Could you check a few things on this model? Use its own coordinates, in mm. A direction names the side the tool comes from. Give positions to 0.01 mm unless a question says otherwise; leave off trailing zeros. Write each loop counter-clockwise with the first axis right and the second up, starting at its lowest first coordinate (ties: lowest second). Pieces come first, ordered by that corner, then holes. Notation, with made-up numbers: (77, 46) - (101, 46) arc R26 ccw to (101, 60) - close; hole circle Ø5 at (51.25, 30). An arc over 180 degrees is marked (long way). Answer in a Markdown table with one row per item.
from build123d import *

# Parameters (mm, degrees)
SKETCH1_W           = 50.8
SKETCH1_H           = 53.975
BOSS_EXTRUDE1_DEPTH = 19.05
FILLET1_R           = 5.08
CUT_EXTRUDE1_DEPTH  = 54.975
SKETCH3_W           = 14.750075479
SKETCH3_H           = 6.35
SKETCH3_W_2         = 17.214026843
CUT_EXTRUDE2_DEPTH  = 19.05
SKETCH4_R           = 3.81
CUT_EXTRUDE3_DEPTH  = 48.625
SKETCH5_W           = 40.64
SKETCH5_H           = 15.24
CUT_EXTRUDE4_DEPTH  = 17.78
FILLET2_R           = 2.54


with BuildPart() as part:
    # Sketch1 → Boss-Extrude1 (new body)
    with BuildSketch(Plane(origin=(0, 0, 0), x_dir=(1, 0, 0), z_dir=(0, 1, 0))):
        with Locations((25.4, 26.9875)):
            Rectangle(SKETCH1_W, SKETCH1_H)
    extrude(amount=BOSS_EXTRUDE1_DEPTH)

    # Fillet1
    fillet1_edges = [part.edges().sort_by_distance(p)[0] for p in [
        (25.4, 19.05, -53.975),
        (25.4, 0, -53.975),
        (25.4, 0, 0),
        (25.4, 19.05, 0),
    ]]
    fillet(fillet1_edges, radius=FILLET1_R)

    # Sketch2 → Cut-Extrude1 (cut, through all)
    with BuildSketch(Plane.XY):
        with BuildLine():
            Line((50.8, 19.05), (37.417396167, 19.05))
            Line((37.417396167, 19.05), (37.417396167, 13.97))
            ThreePointArc((37.417396167, 13.97), (43.3705, 16.9545), (49.323603833, 13.97))
            Line((49.323603833, 13.97), (50.8, 13.97))
            Line((50.8, 13.97), (50.8, 19.05))
        make_face()
        with BuildLine():
            Line((50.8, 13.97), (49.323603833, 13.97))
            ThreePointArc((49.323603833, 13.97), (50.421246598, 11.866888695), (50.8, 9.525))
            Line((50.8, 9.525), (50.8, 13.97))
        make_face()
        with BuildLine():
            ThreePointArc((50.8, 9.525), (50.421246598, 7.183111305), (49.323603833, 5.08))
            Line((49.323603833, 5.08), (50.8, 5.08))
            Line((50.8, 5.08), (50.8, 9.525))
        make_face()
        with BuildLine():
            ThreePointArc((49.323603833, 5.08), (43.3705, 2.0955), (37.417396167, 5.08))
            Line((37.417396167, 5.08), (37.417396167, 0))
            Line((37.417396167, 0), (50.8, 0))
            Line((50.8, 0), (50.8, 5.08))
            Line((50.8, 5.08), (49.323603833, 5.08))
        make_face()
    extrude(amount=-CUT_EXTRUDE1_DEPTH, mode=Mode.SUBTRACT)

    # Sketch3 → Cut-Extrude2 (cut)
    with BuildSketch(Plane(origin=(0, 19.05, 0), x_dir=(1, 0, 0), z_dir=(0, 1, 0))):
        with Locations((44.792433907, 3.175)):
            Rectangle(SKETCH3_W, SKETCH3_H)
        with Locations((46.024409589, 50.8)):
            Rectangle(SKETCH3_W_2, SKETCH3_H)
    extrude(amount=-CUT_EXTRUDE2_DEPTH, mode=Mode.SUBTRACT)

    # Sketch4 → Cut-Extrude3 (cut, through all)
    with BuildSketch(Plane.XY.offset(-6.35)):
        with Locations((43.3705, 9.525)):
            Circle(SKETCH4_R)
    extrude(amount=-CUT_EXTRUDE3_DEPTH, mode=Mode.SUBTRACT)

    # Sketch5 → Cut-Extrude4 (cut)
    with BuildSketch(Plane.ZY):
        with Locations((-26.9875, 9.525)):
            Rectangle(SKETCH5_W, SKETCH5_H)
    extrude(amount=-CUT_EXTRUDE4_DEPTH, mode=Mode.SUBTRACT)

    # Fillet2
    fillet2_edges = [part.edges().sort_by_distance(p)[0] for p in [
        (8.89, 1.905, -47.3075),
        (8.89, 17.145, -47.3075),
        (8.89, 17.145, -6.6675),
        (8.89, 1.905, -6.6675),
    ]]
    fillet(fillet2_edges, radius=FILLET2_R)


solid = part.part
1) Will these pins go through, and if not, where does the flat tip stop? P1, Ø6.5, axis at x = 44, y = 6, coming from the -Z side (3 decimals); P2, Ø4.5, axis at x = 43.37, y = 9.52, coming from the -Z side.
Check values:
| item | result |
|---|---|
| P1 | stops at z = -47.625 |
| P2 | passes through |
2) We'd pull the mould along Z, two halves only. Please class faces 1 (the face through (18.971, 17.522, -1.449)), 2 (the face through (18.97, 17.52, -52.53)), 3 (the face through (46.89, 8.07, -26.7)), 4 (the face through (9.01, 2.63, -7.43)): +Z half, -Z half, draft (parallel to the pull), parting line (faces both ways), or undercut.
Check values:
| item | result |
|---|---|
| face 1 | +Z half |
| face 2 | -Z half |
| face 3 | draft |
| face 4 | undercut |
3) On a 3-axis mill with a long thin cutter (end or side, diameter ignored), from which of +Z, -Z, +X, -X, +Y, -Y can I reach the whole of each face in a straight line? I mean faces 5 (the face through (9, 9, -47.308)), 6 (the face through (47, 11.3, -6.35)), 7 (the face through (47, 11.3, -47.625)), 8 (the face through (0, 1, -27)), 9 (the face through (18, 19.05, -27)). Say none if no direction works.
Check values:
| item | result |
|---|---|
| face 5 | -X |
| face 6 | +Z, +X, +Y, -Y |
| face 7 | -Z, +X, +Y, -Y |
| face 8 | +Z, -Z, -X, +Y, -Y |
| face 9 | +Z, -Z, +X, -X, +Y |
4) Imagine slicing it at C-C (y = 3). List the corners of the cut face in (x, z) for me (3 decimals), then the cut area to 3 significant figures.
Check values:
| item | result |
|---|---|
| outline | (0, -53.53) - (37.417, -53.53) - (37.417, -0.445) - (0, -0.445) - (0, -7.119) - (17.78, -7.119) - (17.78, -46.856) - (0, -46.856) - close; (39.818, -47.625) - (46.923, -47.625) - (46.923, -6.35) - (39.818, -6.35) - close |
| area | 1,570 mm2 |
5) Imagine slicing it at D-D (x = 44.5). List the corners of the cut face in (y, z) for me (3 decimals), then the cut area to 3 significant figures.
Check values:
| item | result |
|---|---|
| outline | (2.182, -47.625) - (5.886, -47.625) - (5.886, -6.35) - (2.182, -6.35) - close; (13.164, -47.625) - (16.868, -47.625) - (16.868, -6.35) - (13.164, -6.35) - close |
| area | 306 mm2 |
6) If I drill on line 1 (Z direction, x = 5.5, y = 11.5) (1 decimal); line 2 (X direction, y = 9.75, z = -52); line 3 (X direction, y = 2.75, z = -22), over which ranges is the centre line in solid material (lowest first)?
Check values:
| item | result |
|---|---|
| line 1 | z = -54 to -47.3, -6.7 to 0 |
| line 2 | x = 0 to 37.42 |
| line 3 | x = 17.78 to 37.42, 40.32 to 46.42 |
